Part model, mm, in its own coordinate system. Coordinates: 2 decimals unless noted, no trailing zeros. Loops run counter-clockwise (first coordinate to the right, second up) from the corner with the lowest first, then second, coordinate; pieces in that order, holes last. Notation, with made-up numbers: (-8.5, 49) - (35.5, 49) arc R14 cw to (35.5, 62) - close; hole circle Ø6 at (34.5, 75). An arc over 180 degrees is marked (long way). Answer as CSV lines item,"result".
Autodesk Inventor part; units mm, degrees
ref_plane "metal_XY" through (0, 0, 0) normal (0, 1, 0) x (1, 0, 0)
ref_plane "metal_YZ" through (0, 0, 0) normal (1, 0, 0) x (0, 0, -1)
ref_plane "metal_ZX" through (0, 0, 0) normal (0, 0, -1) x (0, 1, 0)
sketch "Sketch_7" plane through (0, 0, 7.8994) normal (0, 0, 1) x (1, 0, 0)
  line L0 (-10.8712, 1.3208) -> (10.8712, 1.3208)
  line L1 (10.8712, 1.3208) -> (10.8712, 2.9972)
  line L2 (10.8712, 2.9972) -> (-10.8712, 2.9972)
  line L3 (-10.8712, 2.9972) -> (-10.8712, 1.3208)
extrude "Extrusion1" add sketch "Sketch_7" against normal blind 0.127
sketch "Sketch_11" plane through (-10.9982, 0, 0) normal (1, 0, 0) x (0, 0, -1)
  line L0 (-7.8994, 1.3208) -> (-3.0734, 1.3208)
  arc A0 (-3.0734, 1.3208) -> (-2.8194, 1.5748) centre (-3.0734, 1.5748) ccw
  line L1 (-2.8194, 1.5748) -> (-2.8194, 3.5052)
  arc A1 (-2.8194, 3.5052) -> (-3.0734, 3.7592) centre (-3.0734, 3.5052) ccw
  line L2 (-3.0734, 3.7592) -> (-7.1374, 3.7592)
  arc A2 (-7.1374, 3.7592) -> (-7.3914, 3.5052) centre (-7.1374, 3.5052) ccw
  line L3 (-7.3914, 3.5052) -> (-7.3914, 2.9972)
  line L4 (-7.3914, 2.9972) -> (-7.8994, 2.9972)
  line L5 (-7.8994, 2.9972) -> (-7.8994, 1.3208)
  line L6 (-5.0546, 2.8448) -> (-5.0546, 2.2352)
  line L7 (-5.0546, 2.2352) -> (-4.0386, 2.2352)
  line L8 (-4.0386, 2.2352) -> (-4.0386, 2.8448)
  line L9 (-4.0386, 2.8448) -> (-5.0546, 2.8448)
extrude "Extrusion2" add sketch "Sketch_11" along normal blind 0.127
sketch "Sketch_13" plane through (10.9982, 0, 0) normal (1, 0, 0) x (0, 0, -1)
  line L0 (-7.8994, 1.3208) -> (-3.0734, 1.3208)
  arc A0 (-3.0734, 1.3208) -> (-2.8194, 1.5748) centre (-3.0734, 1.5748) ccw
  line L1 (-2.8194, 1.5748) -> (-2.8194, 3.5052)
  arc A1 (-2.8194, 3.5052) -> (-3.0734, 3.7592) centre (-3.0734, 3.5052) ccw
  line L2 (-3.0734, 3.7592) -> (-7.1374, 3.7592)
  arc A2 (-7.1374, 3.7592) -> (-7.3914, 3.5052) centre (-7.1374, 3.5052) ccw
  line L3 (-7.3914, 3.5052) -> (-7.3914, 2.9972)
  line L4 (-7.3914, 2.9972) -> (-7.8994, 2.9972)
  line L5 (-7.8994, 2.9972) -> (-7.8994, 1.3208)
  line L6 (-5.0546, 2.8448) -> (-5.0546, 2.2352)
  line L7 (-5.0546, 2.2352) -> (-4.0386, 2.2352)
  line L8 (-4.0386, 2.2352) -> (-4.0386, 2.8448)
  line L9 (-4.0386, 2.8448) -> (-5.0546, 2.8448)
extrude "Extrusion3" add sketch "Sketch_13" against normal blind 0.127
sketch "Sketch_17" plane through (0, 0, 0) normal (1, 0, 0) x (0, 1, 0)
  line L0 (8.128, 8.9027) -> (2.9972, 7.8994)
  line L1 (2.9972, 7.8994) -> (2.9972, 7.7726)
  line L2 (2.9972, 7.7726) -> (8.1519, 8.7806)
  line L3 (8.1519, 8.7806) -> (8.128, 8.9027)
extrude "Extrusion4" add sketch "Sketch_17" along normal mid plane 21.336
sketch "Sketch_18" plane through (0, 0, 7.6454) normal (0, 0, 1) x (1, 0, 0)
  line L0 (-11.1252, 8.4328) -> (-11.1252, 2.9972)
  line L1 (-11.1252, 2.9972) -> (-10.6172, 2.9972)
  line L2 (-10.6172, 2.9972) -> (-10.6172, 8.0772)
  line L3 (-10.6172, 8.0772) -> (-10.1092, 8.0772)
  line L4 (-10.1092, 8.0772) -> (-8.78, 4.4254)
  line L5 (-8.78, 4.4254) -> (-8.78, 2.9972)
  line L6 (-8.78, 2.9972) -> (8.78, 2.9972)
  line L7 (8.78, 2.9972) -> (8.78, 4.4254)
  line L8 (8.78, 4.4254) -> (10.1092, 8.0772)
  line L9 (10.1092, 8.0772) -> (10.6172, 8.0772)
  line L10 (10.6172, 8.0772) -> (10.6172, 2.9972)
  line L11 (10.6172, 2.9972) -> (11.1252, 2.9972)
  line L12 (11.1252, 2.9972) -> (11.1252, 8.4328)
  line L13 (11.1252, 8.4328) -> (-11.1252, 8.4328)
extrude "Extrusion5" cut sketch "Sketch_18" along normal blind 2.794
ref_plane "metal_XY" through (0, 0, 0) normal (0, 1, 0) x (1, 0, 0)
ref_plane "metal_YZ" through (0, 0, 0) normal (1, 0, 0) x (0, 0, -1)
ref_plane "metal_ZX" through (0, 0, 0) normal (0, 0, -1) x (0, 1, 0)
properties part number "UB16NKG015F-NR"
Q1. Saw through at B-B (z = 5.5). Give the cut face in (x, y), then the cut area to 3 significant figures.
Results:
outline,"(-11, 1.32) - (-10.87, 1.32) - (-10.87, 3.76) - (-11, 3.76) - close; (10.87, 1.32) - (11, 1.32) - (11, 3.76) - (10.87, 3.76) - close"
area,"0.619 mm^2"
Q2. Saw through at A-A (y = 2.5). Give the cut face in (x, z), then the cut area to 3 significant figures.
Results:
outline,"(-11, 2.82) - (-10.87, 2.82) - (-10.87, 4.04) - (-11, 4.04) - close; (-11, 5.05) - (-10.87, 5.05) - (-10.87, 7.77) - (10.87, 7.77) - (10.87, 5.05) - (11, 5.05) - (11, 7.9) - (-11, 7.9) - close; (10.87, 2.82) - (11, 2.82) - (11, 4.04) - (10.87, 4.04) - close"
area,"3.79 mm^2"
Q3. Saw through at C-C (y = 6.25). Give the cut face in (x, z), then the cut area to 3 significant figures.
Results:
outline,"(-10.62, 8.41) - (-9.44, 8.41) - (-9.44, 8.54) - (-10.62, 8.54) - close; (9.44, 8.41) - (10.62, 8.41) - (10.62, 8.54) - (9.44, 8.54) - close"
area,"0.297 mm^2"
Q4. Flat gauge pins, fed straight in: pin 1 (0.5 mm diameter, centred on x = 3, y = 2.5, fed in from +Z); pin 2 (1.8 mm diameter, centred on x = 5, y = 2, fed in from -Z); pin 3 (0.6 mm diameter, centred on y = 5.5, z = 8.5, fed in from +X); pin 4 (1 mm diameter, centred on x = 1.5, y = 4.5, fed in from -Z). Where does each tip first touch, or does it go through?
Results:
pin 1,"stops at z = 7.9"
pin 2,"stops at z = 7.77"
pin 3,"stops at x = 10.62"
pin 4,"passes through"
